For this review, take the finished solid that the model builds, in its own axes (mm). Coordinates: 2 decimals unless noted, no trailing zeros. Write each loop counter-clockwise with the first axis right and the second up, starting at its lowest first coordinate (ties: lowest second). Pieces come first, ordered by that corner, then holes. Notation, with made-up numbers: (18.5, 24.5) - (36.5, 24.5) arc R25 ccw to (36.5, 59.5) - close; hole circle Ø8 at (84.25, -14.5). An arc over 180 degrees is marked (long way). Use one line per item in the form item = value. Start each with the question number.
1) We need section D-D (x = 22.5). Give the boundary of the cut face in (y, z).
2) We need section C-C (y = 2). Count the separate pieces of the cut face and the enclosed holes in it, plus the area to 3 significant figures.
3) We need section A-A (z = -36.5). Give the boundary of the cut face in (x, y), plus the area to 3 significant figures.
4) We need section B-B (x = 10). Give the boundary of the cut face in (y, z).
5) For L1, parallel to Z at x = 22, y = 2.05; L2, parallel to Z at x = 65, y = 1.85; L3, parallel to Z at x = 37.5, y = 0.95, list the stretches that pass through material, from the lowest coordinate up. Write a range as from..to.
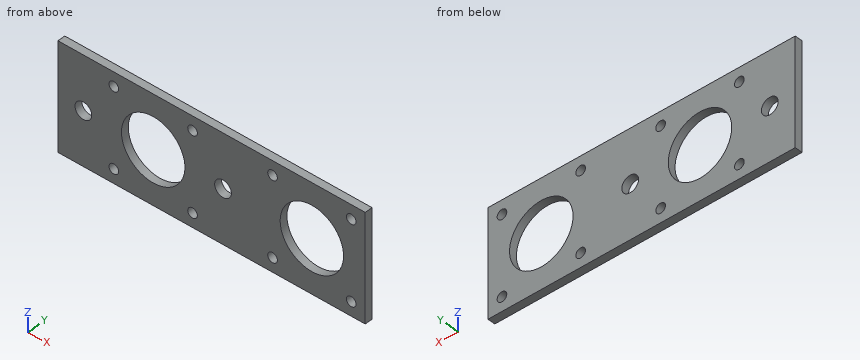
```python
from build123d import *

# Parameters (mm, degrees)
SKETCH_1_W      = 75
SKETCH_1_H      = 42
EXTRUDE_1_DEPTH = 3
HOLE_WIZARD_1_D = 3.8
HOLE_WIZARD_2_D = 6.6
HOLE_WIZARD_3_D = 25
EXTRUDE_2_DEPTH = 3
HOLE_WIZARD_4_D = 3.8
HOLE_WIZARD_5_D = 25


with BuildPart() as part:
    # 草图1 → 凸台-拉伸1 (new body)
    with BuildSketch(Plane(origin=(0, 0, 0), x_dir=(1, 0, 0), z_dir=(0, 1, 0))):
        with Locations((37.5, 21)):
            Rectangle(SKETCH_1_W, SKETCH_1_H)
    extrude(amount=EXTRUDE_1_DEPTH)

    # 孔1 (through all)
    with Locations(Plane(origin=(0, 3, 0), x_dir=(1, 0, 0), z_dir=(0, 1, 0))):
        with Locations((22, 36.5), (53, 36.5), (53, 5.5), (22, 5.5)):
            Hole(HOLE_WIZARD_1_D / 2)

    # 孔2 (through all)
    with Locations(Plane(origin=(0, 3, 0), x_dir=(1, 0, 0), z_dir=(0, 1, 0))):
        with Locations((10, 21), (65, 21)):
            Hole(HOLE_WIZARD_2_D / 2)

    # 孔3 (through all)
    with Locations(Plane(origin=(0, 3, 0), x_dir=(1, 0, 0), z_dir=(0, 1, 0))):
        with Locations((37.5, 21)):
            Hole(HOLE_WIZARD_3_D / 2)

    # 草图9 → 凸台-拉伸2 (add)
    with BuildSketch(Plane(origin=(0, 3, 0), x_dir=(1, 0, 0), z_dir=(0, 1, 0))):
        Polygon((121, 42), (75, 42), (75, 21), (75, 0), (121, 0), align=None)
    extrude(amount=-EXTRUDE_2_DEPTH)

    # 孔4 (through all)
    with Locations(Plane(origin=(0, 3, 0), x_dir=(1, 0, 0), z_dir=(0, 1, 0))):
        with Locations((84.5, 36.5), (115.5, 36.5), (115.5, 5.5), (84.5, 5.5)):
            Hole(HOLE_WIZARD_4_D / 2)

    # 孔5 (through all)
    with Locations(Plane(origin=(0, 3, 0), x_dir=(1, 0, 0), z_dir=(0, 1, 0))):
        with Locations((100, 21)):
            Hole(HOLE_WIZARD_5_D / 2)


solid = part.part
```
Determined:
q1.outline = (0, -42) - (3, -42) - (3, -38.33) - (0, -38.33) - close; (0, -34.67) - (3, -34.67) - (3, -7.33) - (0, -7.33) - close; (0, -3.67) - (3, -3.67) - (3, 0) - (0, 0) - close
q2.separate_pieces = 1
q2.enclosed_holes = 12
q2.area = 3,940 mm²
q3.outline = (0, 0) - (20.1, 0) - (20.1, 3) - (0, 3) - close; (23.9, 0) - (51.1, 0) - (51.1, 3) - (23.9, 3) - close; (54.9, 0) - (82.6, 0) - (82.6, 3) - (54.9, 3) - close; (86.4, 0) - (113.6, 0) - (113.6, 3) - (86.4, 3) - close; (117.4, 0) - (121, 0) - (121, 3) - (117.4, 3) - close
q3.area = 317 mm²
q4.outline = (0, -42) - (3, -42) - (3, -24.3) - (0, -24.3) - close; (0, -17.7) - (3, -17.7) - (3, 0) - (0, 0) - close
q5.L1 = -42..-38.4, -34.6..-7.4, -3.6..0
q5.L2 = -42..-24.3, -17.7..0
q5.L3 = -42..-33.5, -8.5..0
